```python
from build123d import *

# Parameters (mm, degrees)
SKETCH1_R           = 8.5
BOSS_EXTRUDE1_DEPTH = 35.5
SKETCH3_R           = 7
BOSS_EXTRUDE2_DEPTH = 5
SKETCH5_R           = 5
BOSS_EXTRUDE3_DEPTH = 25
SKETCH2_R           = 4
CUT_EXTRUDE1_DEPTH  = 17


with BuildPart() as part:
    # Sketch1 → Boss-Extrude1 (new body)
    with BuildSketch(Plane(origin=(0, 0, 0), x_dir=(1, 0, 0), z_dir=(0, 1, 0))):
        Circle(SKETCH1_R)
    extrude(amount=BOSS_EXTRUDE1_DEPTH)

    # Sketch3 → Boss-Extrude2 (add)
    with BuildSketch(Plane(origin=(0, 0, 0), x_dir=(-1, 0, 0), z_dir=(0, -1, 0))):
        Circle(SKETCH3_R)
    extrude(amount=BOSS_EXTRUDE2_DEPTH)

    # Sketch5 → Boss-Extrude3 (add)
    with BuildSketch(Plane(origin=(0, -5, 0), x_dir=(-1, 0, 0), z_dir=(0, -1, 0))):
        Circle(SKETCH5_R)
    extrude(amount=BOSS_EXTRUDE3_DEPTH)

    # Sketch2 → Cut-Extrude1 (cut)
    with BuildSketch(Plane(origin=(0, 35.5, 0), x_dir=(1, 0, 0), z_dir=(0, 1, 0))):
        Circle(SKETCH2_R)
    extrude(amount=-CUT_EXTRUDE1_DEPTH, mode=Mode.SUBTRACT)


solid = part.part
```
Verification items for the finished model (mm, model axes). A direction names the side the tool comes from. Round coordinates to 2 decimals unless told otherwise and drop trailing zeros. Write each loop counter-clockwise with the first axis right and the second up, starting at its lowest first coordinate (ties: lowest second). Pieces come first, ordered by that corner, then holes. Notation, with made-up numbers: (84, 66.5) -> (120, 66.5) arc R19 ccw to (120, 77.5) -> close; hole circle Ø5 at (-31, -38). An arc over 180 degrees is marked (long way). Write each question's results on one line, items separated by ' | '. Start each with the question number.
1. Cross-section at D-D (y = 7.5). Enter the section's corners in (x, z), then the cut area to 3 significant figures.
2. Set-up check for faces 1 (the flat face through (0, -30, 0)), 2 (the cylindrical face through (-6.466, -2.465, 2.681)), 3 (the cylindrical face through (-0.867, 27.119, 3.905)): record each of +Z, -Z, +X, -X, +Y, -Y from which the full face is reachable in a straight line by a thin tool's end or side.
3. Cross-section at C-C (y = 29). Enter the section's corners in (x, z), then the cut area to 3 significant figures.
4. Draft check along Z on faces 4 (the flat face through (0, 18.5, 0)), 5 (the cylindrical face through (1.08, -17.32, 4.88)), 6 (the flat face through (4, 35.5, 2)). Enter one of: +Z half, -Z half, draft (parallel to the pull), parting line (faces both ways), or undercut.
5. Material ranges on probe 1 along X at (y, z) = (22.75, 0); probe 2 along Y at (x, z) = (-6.75, -5), recorded low to high. Write a range as from..to.
6. Cross-section at B-B (x = 0). Enter the section's corners in (y, z).
7. Depth check by flat-ended pin: P1, Ø1.5, axis at x = -0.5, z = -1.5, coming from the +Y side; P2, Ø3, axis at x = -1, y = -9.5, coming from the -Z side; P3, Ø1.5, axis at y = -6.5, z = 1.5, coming from the +X side. Enter the tip coordinate at first touch or a pass-through.
8. Cross-section at A-A (z = 0). Enter the section's corners in (x, y).
Solutions:
1) outline: circle Ø17 at (0, 0) | area: 227 mm2
2) face 1: +Z, -Z, +X, -X, -Y | face 2: -Y | face 3: +Y
3) outline: circle Ø17 at (0, 0); hole circle Ø8 at (0, 0) | area: 177 mm2
4) face 4: undercut | face 5: parting line | face 6: draft
5) probe 1: x = -8.5..-4, 4..8.5 | probe 2: y = 0..35.5
6) outline: (-30, -5) -> (-5, -5) -> (-5, -7) -> (0, -7) -> (0, -8.5) -> (35.5, -8.5) -> (35.5, -4) -> (18.5, -4) -> (18.5, 4) -> (35.5, 4) -> (35.5, 8.5) -> (0, 8.5) -> (0, 7) -> (-5, 7) -> (-5, 5) -> (-30, 5) -> close
7) P1: stops at y = 18.5 | P2: stops at z = -5 | P3: stops at x = 4.94
8) outline: (-8.5, 0) -> (-7, 0) -> (-7, -5) -> (-5, -5) -> (-5, -30) -> (5, -30) -> (5, -5) -> (7, -5) -> (7, 0) -> (8.5, 0) -> (8.5, 35.5) -> (4, 35.5) -> (4, 18.5) -> (-4, 18.5) -> (-4, 35.5) -> (-8.5, 35.5) -> close
